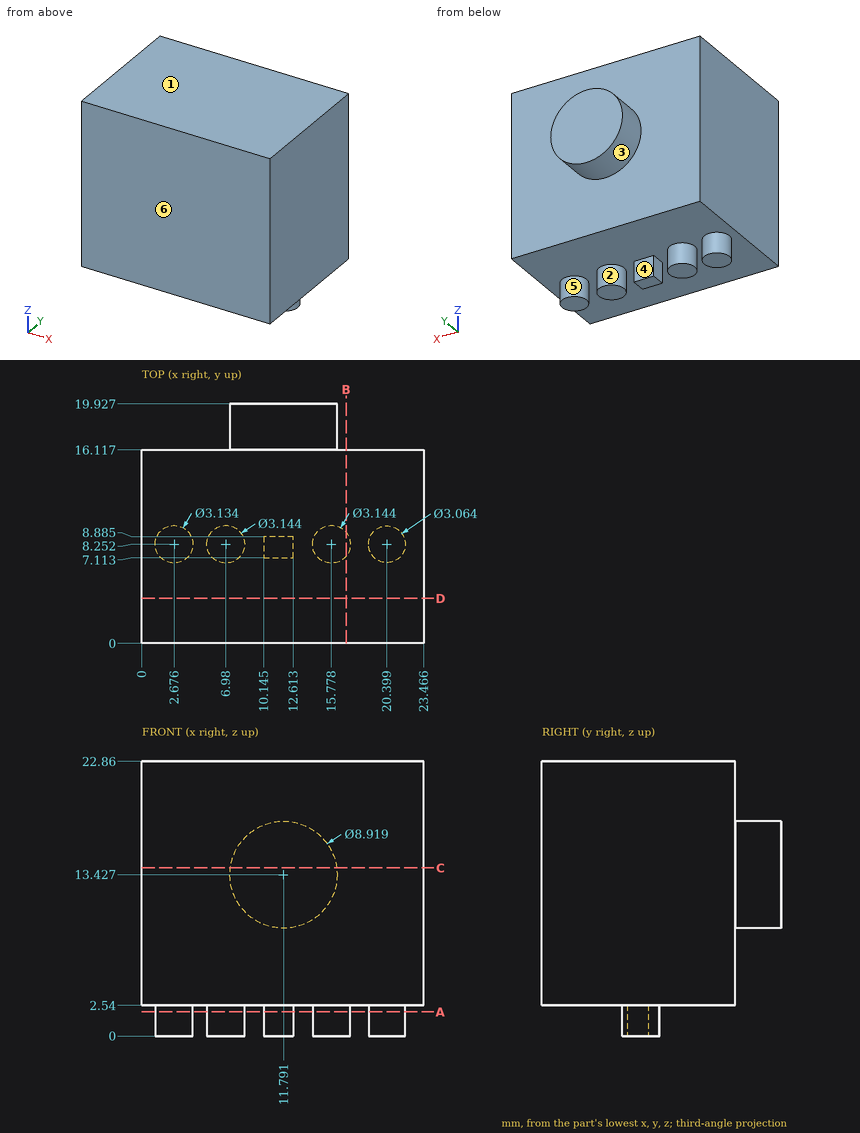
Study the drawing (mm; zero at the part's minimum x, y, z) and answer. A direction names the side the tool comes from. Round coordinates to 2 decimals unless told otherwise and drop trailing zeros. Write each loop counter-clockwise with the first axis right and the second up, starting at its lowest first coordinate (ties: lowest second). Pieces come first, ordered by that corner, then holes. Notation, with made-up numbers: (21.5, 71) - (28.5, 71) arc R29 ccw to (28.5, 99) - close; hole circle Ø8 at (-5.5, -1). An arc over 180 degrees is marked (long way). Use a Markdown table: item, result. Add a question column.
1. Consider line 1 (Y direction, x = 18, z = 20.25); line 2 (Z direction, x = 11, y = 2.75); line 3 (Z direction, x = 13, y = 17.5) (1 decimal). Determine where each line is inside the solid, lowest interval first.
2. The part is cut by section D-D (y = 3.75). Write down the section's boundary in (x, z).
3. The part is cut by section B-B (x = 17). Write down the section's boundary in (y, z).
4. Flat-ended cylindrical pins translate along their axes: P1, Ø0.7, axis at x = 12, z = 1, coming from the -Y side; P2, Ø6, axis at x = 3, y = 15, coming from the -Z side; P3, Ø0.5, axis at y = 7.5, z = 1, coming from the +X side. Find the tip coordinate at first contact, or state that the pin passes through.
5. A tool of negligible diameter and unlimited length cuts with its end or side. For the marked faces 4, 5 and 6, from which of +Z, -Z, +X, -X, +Y, -Y can it reach the whole face along a straight path? Write none if from no direction.
6. For a pull along X with two mould halves and no side action, classify the marked faces 1, 2 and 3 as +X half, -X half, draft (parallel to the pull), parting line (faces both ways), or undercut.
7. The part is cut by section A-A (z = 2). Write down the section's boundary in (x, y) (1 decimal).
8. The part is cut by section C-C (z = 14). Write down the section's boundary in (x, y), and give its area (3 significant figures).
Reported:
| question | item | result |
|---|---|---|
| 1 | line 1 | 0 to 16.12 |
| 1 | line 2 | 2.54 to 22.86 |
| 1 | line 3 | 9.1 to 17.7 |
| 2 | outline | (0, 2.54) - (23.47, 2.54) - (23.47, 22.86) - (0, 22.86) - close |
| 3 | outline | (0, 2.54) - (7.26, 2.54) - (7.26, 0) - (9.24, 0) - (9.24, 2.54) - (16.12, 2.54) - (16.12, 22.86) - (0, 22.86) - close |
| 4 | P1 | y = 7.11 |
| 4 | P2 | z = 2.54 |
| 4 | P3 | x = 21.85 |
| 5 | face 4 | -Z, +Y |
| 5 | face 5 | -Z |
| 5 | face 6 | +Z, -Z, +X, -X, -Y |
| 6 | face 1 | draft |
| 6 | face 2 | undercut |
| 6 | face 3 | parting line |
| 7 | outline | circle Ø3.1 at (2.7, 8.3); circle Ø3.1 at (7, 8.3); (10.1, 7.1) - (12.6, 7.1) - (12.6, 8.9) - (10.1, 8.9) - close; circle Ø3.1 at (15.8, 8.3); circle Ø3.1 at (20.4, 8.3) |
| 8 | outline | (0, 0) - (23.47, 0) - (23.47, 16.12) - (16.21, 16.12) - (16.21, 19.93) - (7.37, 19.93) - (7.37, 16.12) - (0, 16.12) - close |
| 8 | area | 412 mm^2 |
